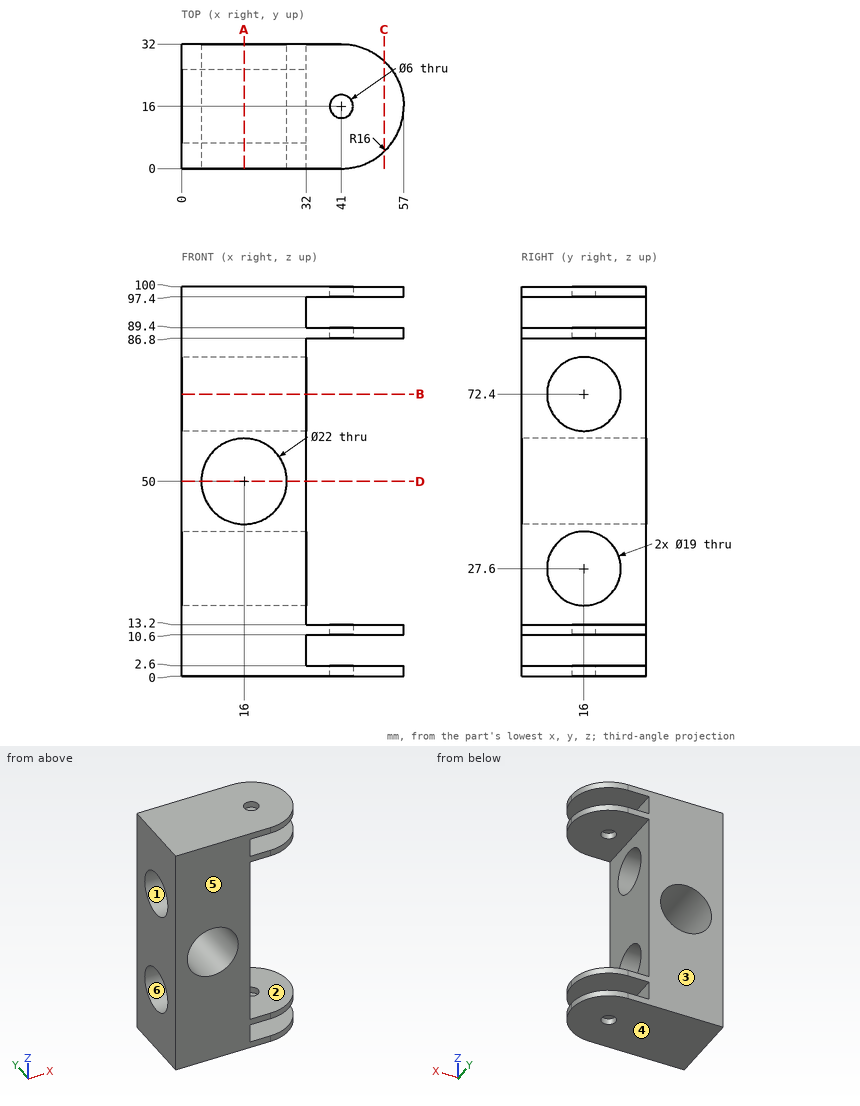
Design review of the part shown in the three views and the two pictorial views. Dimensions are in mm from the part's minimum x, y and z. A direction names the side the tool comes from. Round coordinates to 2 decimals unless told otherwise and drop trailing zeros. Write each loop counter-clockwise with the first axis right and the second up, starting at its lowest first coordinate (ties: lowest second). Pieces come first, ordered by that corner, then holes. Notation, with made-up numbers: (-26, 58.5) - (-13, 58.5) arc R38 cw to (-13, 97.5) - close; hole circle Ø5 at (58.25, 8.25). An arc over 180 degrees is marked (long way). Write item = value, one per line. Start each with the question number.
1. Consider section A-A on x = 16. State the section outline as (y, z) points, plus the area to 3 significant figures.
2. For pin 1 Ø17.5 at (x, z) = (16, 50) entering from -Y; pin 2 Ø4 at (y, z) = (22, 95) entering from +X, all flat-tipped, find the tip position at first contact; note any pin that passes through.
3. Consider section D-D on z = 50. State the section outline as (x, y) points, plus the area to 3 significant figures.
4. Draft analysis for pull direction Y (two halves, no side actions). For the marked faces 3, 4, 5 and 6, state which applies: released by +Y, released by -Y, zero draft, split by the parting line, or undercut.
5. For the marked faces 1 and 2, list the 3-axis set-ups (+Z, -Z, +X, -X, +Y, -Y) from which the entire face can be reached by the end or side of a thin tool; tool diameter is ignored.
6. Consider section B-B on z = 72.4. State the section outline as (x, y) points.
7. Wall thickness on L1, parallel to Z at x = 33.5, y = 12; L2, parallel to Y at x = 41, z = 11; L3, parallel to Z at x = 18, y = 18: over which ranges is each line inside the solid? List them lowest first.
8. Consider section C-C on x = 52. State the section outline as (y, z) points.
Evaluation:
q1.outline = (0, 0) - (32, 0) - (32, 39) - (0, 39) - close; (0, 61) - (32, 61) - (32, 100) - (0, 100) - close; hole circle Ø19 at (16, 27.6); hole circle Ø19 at (16, 72.4)
q1.area = 1,930 mm2
q2.pin_1 = through
q2.pin_2 = 32
q3.outline = (0, 0) - (5, 0) - (5, 32) - (0, 32) - close; (27, 0) - (32, 0) - (32, 32) - (27, 32) - close
q3.area = 320 mm2
q4.face_3 = released by +Y
q4.face_4 = zero draft
q4.face_5 = released by -Y
q4.face_6 = undercut
q5.face_1 = +X, -X
q5.face_2 = +X, +Y, -Y
q6.outline = (0, 0) - (32, 0) - (32, 6.5) - (0, 6.5) - close; (0, 25.5) - (32, 25.5) - (32, 32) - (0, 32) - close
q7.L1 = 0 to 2.6, 10.6 to 13.2, 86.8 to 89.4, 97.4 to 100
q7.L2 = 0 to 13, 19 to 32
q7.L3 = 0 to 18.31, 36.89 to 39.18, 60.82 to 63.11, 81.69 to 100
q8.outline = (4.38, 0) - (27.62, 0) - (27.62, 2.6) - (4.38, 2.6) - close; (4.38, 10.6) - (27.62, 10.6) - (27.62, 13.2) - (4.38, 13.2) - close; (4.38, 86.8) - (27.62, 86.8) - (27.62, 89.4) - (4.38, 89.4) - close; (4.38, 97.4) - (27.62, 97.4) - (27.62, 100) - (4.38, 100) - close
